Autodesk Fusion 360 part; units mm, degrees
sketch "Sketch1" plane through (0, 0, 0) normal (0, 0, 1) x (1, 0, 0)
  circle A0 centre (0, 0) radius 12.5
  circle A1 centre (0, 0) radius 7.5
  circle A2 centre (-35, 0) radius 5
  circle A3 centre (35, 0) radius 5
  line L0 (-60, 0) -> (60, 0) construction
  line L1 (-35, 0) -> (-35, 14) construction
  line L2 (-35, 14) -> (-35, -13) construction
  line L3 (35, 0) -> (35, 14) construction
  line L4 (35, 14) -> (35, -13) construction
  line L5 (-36.4286, -9.8974) -> (-2.1429, -14.8461)
  line L6 (36.4286, -9.8974) -> (2.1429, -14.8461)
  line L7 (36.4286, 9.8974) -> (2.1429, 14.8461)
  line L8 (-36.4286, 9.8974) -> (-2.1429, 14.8461)
  arc A4 (-35, 10) -> (-35, -10) centre (-35, 0) ccw
  arc A5 (35, -10) -> (35, 10) centre (35, 0) ccw
  arc A6 (-2.1429, -14.8461) -> (2.1429, -14.8461) centre (0, 0) ccw
  arc A7 (2.1429, 14.8461) -> (-2.1429, 14.8461) centre (0, 0) ccw
  dimension "d1" = 30
  dimension "d2" = 25
  dimension "d3" = 15
  dimension "d4" = 10
  dimension "d5" = 10
  dimension "d6" = 20
  dimension "d7" = 20
  dimension "d8" = 35
  dimension "d9" = 35
extrude "Extrude1" add sketch "Sketch1" along normal blind 5 contours L5 L6 L7 L8 A4 A5 A6 A7
sketch "Sketch2" plane through (0, 0, 0) normal (0, 0, 1) x (1, 0, 0)
  circle A0 centre (0, 0) radius 12.5
  circle A1 centre (0, 0) radius 7.5
  dimension "d12" = 25
  dimension "d13" = 15
extrude "Extrude2" add sketch "Sketch2" along normal blind 30
sketch "Sketch6" plane through (0, 0, 0) normal (0, 1, 0) x (1, 0, 0)
  line L0 (-10, -5) -> (-25, -5)
  line L1 (-25, -5) -> (-10, -30)
  line L2 (-10, -30) -> (-10, -5)
  line L3 (10, -5) -> (25, -5)
  line L4 (25, -5) -> (10, -30)
  line L5 (10, -30) -> (10, -5)
  line L6 (-36.4286, -5) -> (-2.1429, -5)
  line L7 (2.1429, -5) -> (36.4286, -5)
  dimension "d27" = 10
  dimension "d28" = 10
  dimension "d29" = 15
  dimension "d30" = 15
  dimension "d31" = 25
extrude "Extrude4" add sketch "Sketch6" along normal blind 2.5 and the other way blind 2.5
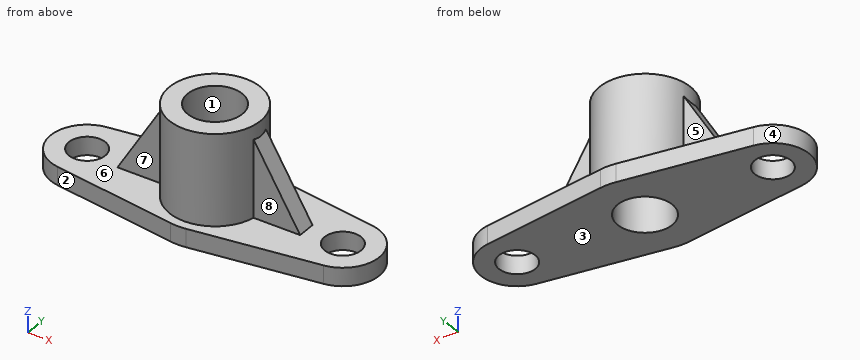
The listing builds one solid part. Answer for the finished solid, in the listing's coordinates (mm). Face numbers are marked on the shaded views. A direction names the side the tool comes from. Round coordinates to 2 decimals unless told otherwise and drop trailing zeros. Loops run counter-clockwise (first coordinate to the right, second up) from the corner with the lowest first, then second, coordinate; pieces in that order, holes last. Notation, with made-up numbers: M 64,39 L 115,39 A35 ccw 115,75 Z; hole C 3.25,32 d8. An arc over 180 degrees is marked long. Write each question's results on one line, items separated by ' | '. Start each with the question number.
1) Which of the six approach directions +Z, -Z, +X, -X, +Y, -Y give full straight-line access (tool end or side, diameter ignored) to the marked faces 4, 5, 6, 7 and 8?
2) Each of these flat-tipped pins is pushed along its axis until it touches: pin 1 (5 mm diameter, centred on x = 17.5, z = 11.5, fed in from +Y); pin 2 (2 mm diameter, centred on x = -16.5, y = 8, fed in from +Z); pin 3 (6.5 mm diameter, centred on x = 17, z = 19, fed in from -Y). Where does it stop, or does it pass through?
3) Find section C-C on z = 9.75. Write down the section's boundary in (x, y), plus the area to 3 significant figures.
4) Find section D-D on x = -20.5. Write down the section's boundary in (y, z).
5) Find section A-A on x = 0. Write down the section's boundary in (y, z), plus the area to 3 significant figures.
6) Determine the mould class of the marked faces 1, 2 and 3 for opening direction X: pulls with the +X half, pulls with the -X half, needs draft (parallel to the pull), parting line crosses it, or undercut.
7) Straight lines are drawn through the part: probe 1 along Y at (x, z) = (0, 20); probe 2 along X at (y, z) = (4.5, 2.25); probe 3 along X at (y, z) = (0.5, 4.75). For each, find the intervals that lie inside material, in ascending order.
8) Find section B-B on y = 0. Write down the section's boundary in (x, z).
Final values:
1) face 4: +Z, -Z, -X | face 5: +Z, -X, +Y | face 6: +Z | face 7: +Z, -X, -Y | face 8: +Z, +X, -Y
2) pin 1: y = 2.5 | pin 2: z = 5 | pin 3: y = -2.5
3) outline: M -22.15,-2.5 L -12.25,-2.5 A12.5 ccw 12.25,-2.5 L 22.15,-2.5 L 22.15,2.5 L 12.25,2.5 A12.5 ccw -12.25,2.5 L -22.15,2.5 Z; hole C 0,0 d15 | area: 411 mm²
4) outline: M -12.2,0 L 12.2,0 L 12.2,5 L 2.5,5 L 2.5,12.5 L -2.5,12.5 L -2.5,5 L -12.2,5 Z
5) outline: M -15,0 L -7.5,0 L -7.5,30 L -12.5,30 L -12.5,5 L -15,5 Z; M 7.5,0 L 15,0 L 15,5 L 12.5,5 L 12.5,30 L 7.5,30 Z | area: 325 mm²
6) face 1: undercut | face 2: pulls with the -X half | face 3: needs draft
7) probe 1: -12.5 to -7.5, 7.5 to 12.5 | probe 2: -43.93 to -37.18, -32.82 to -6, 6 to 32.82, 37.18 to 43.93 | probe 3: -44.99 to -39.97, -30.03 to -7.48, 7.48 to 30.03, 39.97 to 44.99
8) outline: M -45,0 L -40,0 L -40,5 L -45,5 Z; M -30,0 L -7.5,0 L -7.5,30 L -12.5,30 L -12.5,25.83 L -25,5 L -30,5 Z; M 7.5,0 L 30,0 L 30,5 L 25,5 L 12.5,25.83 L 12.5,30 L 7.5,30 Z; M 40,0 L 45,0 L 45,5 L 40,5 Z
